Geometry check sheet. Reference: drawing and pictorial views, mm from the part's lowest x, y, z. A direction names the side the tool comes from. Round coordinates to 2 decimals unless told otherwise and drop trailing zeros. Loops run counter-clockwise (first coordinate to the right, second up) from the corner with the lowest first, then second, coordinate; pieces in that order, holes last. Notation, with made-up numbers: (15, 40) - (55, 40) arc R33 ccw to (55, 78) - close; hole circle Ø8 at (16.25, 23.25). An arc over 180 degrees is marked (long way). Return JSON: item names as keys, results as strings.
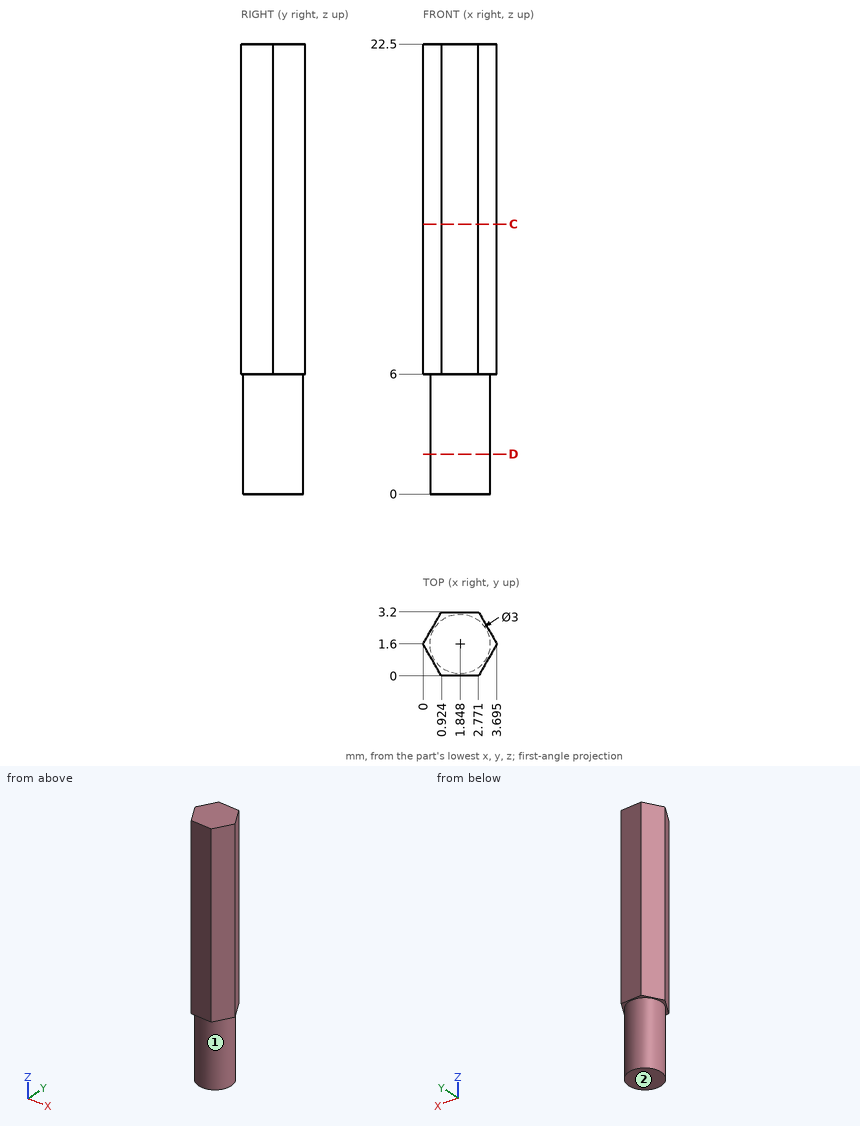
Q1. Tool access check on the marked faces 1 and 2. Record the directions out of +Z, -Z, +X, -X, +Y, -Y that give a thin tool (end or side, any length) a straight path to the whole face; none if there is none.
Answer key:
{"face 1": "-Z", "face 2": "-Z, +X, -X, +Y, -Y"}
Q2. Depth check by flat-ended pin: P1, Ø1.5, axis at y = 0.5, z = 17.5, coming from the -X side. Enter the tip coordinate at first touch or a pass-through.
Answer key:
{"P1": "stops at x = 0.2"}
Q3. Scan lines: probe 1 along Z at (x, y) = (0.55, 2.45); probe 2 along X at (y, z) = (0.8, 8) (1 decimal); probe 3 along X at (y, z) = (2.15, 14.5). Record each from-to range of solid material in increasing order. Write a range as [from, to].
Answer key:
{"probe 1": "z = [6, 22.5]", "probe 2": "x = [0.5, 3.2]", "probe 3": "x = [0.32, 3.38]"}
Q4. Sectioned sample at D-D (z = 2). Enter the section's corners in (x, y).
Answer key:
{"outline": "circle Ø3 at (1.85, 1.6)"}
Q5. Sectioned sample at C-C (z = 13.5). Enter the section's corners in (x, y) (1 decimal).
Answer key:
{"outline": "(0, 1.6) - (0.9, 0) - (2.8, 0) - (3.7, 1.6) - (2.8, 3.2) - (0.9, 3.2) - close"}
